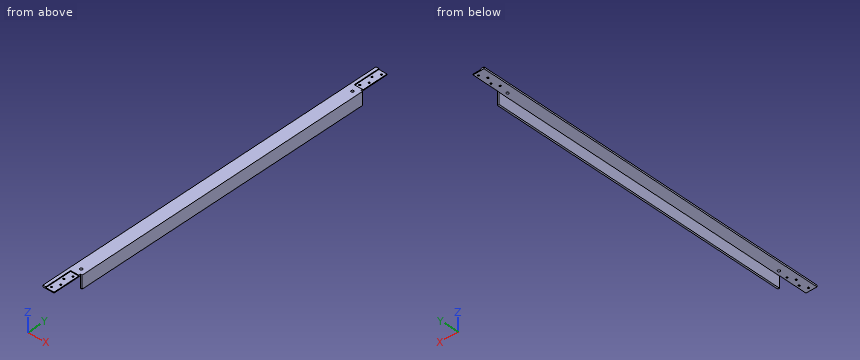
```python
from build123d import *

# Parameters (mm, degrees)
F1_DEPTH = 685.8
F2_W     = 30.95625
F2_H     = 101.6
F2_R     = 3.175
F3_DEPTH = 3.175
F4_DEPTH = 49.2262
F5_D     = 6.35
F7_D     = 9.525


with BuildPart() as f1:
    # F0 (on Front) → F1 (new body, symmetric)
    with BuildSketch(Plane.XZ):
        Polygon((18.2626, -24.6126), (24.6126, -24.6126), (24.6126, 24.6126), (-24.6126, 24.6126), (-24.6126, 18.2626), (18.2626, 18.2626), align=None)
    extrude(amount=F1_DEPTH, both=True)

    # F2 (on face) → F3 (cut)
    with BuildSketch(Plane.XY.offset(24.6126)):
        with Locations((1.990725, -635)):
            Rectangle(F2_W, F2_H)
        with Locations((-3.9624, -673.1)):
            Circle(F2_R, mode=Mode.SUBTRACT)
        with Locations((-3.9624, -622.3)):
            Circle(F2_R, mode=Mode.SUBTRACT)
        with Locations((7.94385, -647.7)):
            Circle(F2_R, mode=Mode.SUBTRACT)
        with Locations((7.94385, -596.9)):
            Circle(F2_R, mode=Mode.SUBTRACT)
        with Locations((1.990725, 635)):
            Rectangle(F2_W, F2_H)
        with Locations((-3.9624, 596.9)):
            Circle(F2_R, mode=Mode.SUBTRACT)
        with Locations((-3.9624, 647.7)):
            Circle(F2_R, mode=Mode.SUBTRACT)
        with Locations((7.94385, 622.3)):
            Circle(F2_R, mode=Mode.SUBTRACT)
        with Locations((7.94385, 673.1)):
            Circle(F2_R, mode=Mode.SUBTRACT)
    extrude(amount=-F3_DEPTH, mode=Mode.SUBTRACT)

    # F2 (on face) → F4 (cut, through all)
    with BuildSketch(Plane.XY.offset(24.6126)):
        Polygon((17.46885, 577.85), (24.6126, 577.85), (24.6126, 685.8), (17.46885, 685.8), (17.46885, 584.2), align=None)
        Polygon((17.46885, -685.8), (24.6126, -685.8), (24.6126, -577.85), (17.46885, -577.85), (17.46885, -584.2), align=None)
    extrude(amount=-F4_DEPTH, mode=Mode.SUBTRACT)

    # F5 (through all)
    with Locations(Plane.XY.offset(24.6126)):
        with Locations((7.94385, -647.7), (-3.9624, -673.1), (-3.9624, -622.3), (7.94385, -596.9), (-3.9624, 647.7), (7.94385, 673.1), (7.94385, 622.3), (-3.9624, 596.9)):
            Hole(F5_D / 2)

    # F7 (through all)
    with Locations(Plane.XY.offset(24.6126)):
        with Locations((3.284499, -558.8), (3.284499, 558.8)):
            Hole(F7_D / 2)


solid = f1.part
```
Input: part model. Units: mm. Frame: model coordinates. Give positions to 0.01 mm unless a question says otherwise; leave off trailing zeros. Loops run counter-clockwise (first coordinate to the right, second up) from the corner with the lowest first, then second, coordinate; pieces in that order, holes last. Notation, with made-up numbers: M 40.5,49 L 70.5,49 A29 cw 70.5,78 Z; hole C -0.5,-33.75 d1. An arc over 180 degrees is marked long. Answer as CSV lines item,"result". Start each with the question number.
1. Line query: L1, parallel to X at y = -622.3, z = 19.6; L2, parallel to X at y = 622.3, z = 20.5; L3, parallel to Z at x = -8, y = 302.5. Output: solid intervals per line, ascending.
2. Section B-B on z = 9.5. Return loops of the section in (x, y), plus the area to 3 significant figures.
3. Section A-A on y = -297. Return loops of the section in (x, z).
4. Pin query (flat end, axial travel): P1, Ø1, axis at x = 2, y = 78.5, coming from the -Z side; P2, Ø2, axis at x = 21.5, z = -7.5, coming from the -Y side; P3, Ø3.5, axis at y = -628.5, z = 23.5, coming from the +X side. Return the tip coordinate at first contact, or that it passes through.
Computed values:
1,L1,"x = -24.61 to -7.14, -0.79 to 17.47"
1,L2,"x = -24.61 to 4.77, 11.12 to 17.47"
1,L3,"z = 18.26 to 24.61"
2,outline,"M 18.26,-577.85 L 24.61,-577.85 L 24.61,577.85 L 18.26,577.85 Z"
2,area,"7,340 mm²"
3,outline,"M -24.61,18.26 L 18.26,18.26 L 18.26,-24.61 L 24.61,-24.61 L 24.61,24.61 L -24.61,24.61 Z"
4,P1,"stops at z = 18.26"
4,P2,"stops at y = -577.85"
4,P3,"stops at x = -13.49"
